Geometry: see drawing. Coordinates: mm, zero at the bounding-box minimum. A direction names the side the tool comes from. Give positions to 0.01 mm unless a question says otherwise; leave off trailing zeros. Order: outer loops, then holes, each group sorted by start corner. A loop starts at its lowest first (then second) coordinate and runs counter-clockwise, first axis right, second up. Notation, with made-up numbers: M 50.5,29 L 94.5,29 A8 cw 94.5,39 Z; hole C 63.5,-29 d4. An arc over 180 degrees is marked long. Return JSON: item names as keys, results as strings.
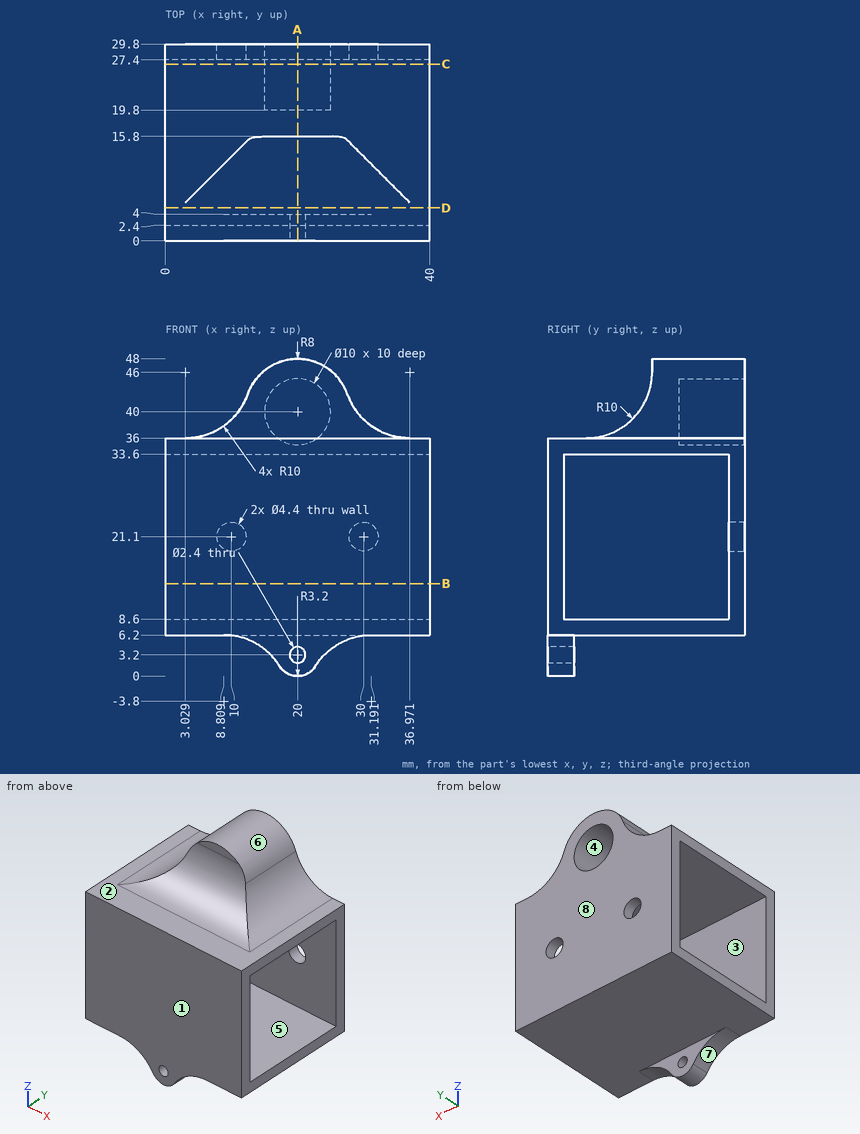
1. Section query A-A (x = 20). Return loops of the section in (y, z).
Evaluation:
{"outline": "M 0,0 L 4,0 L 4,2 L 0,2 Z; M 0,4.4 L 4,4.4 L 4,6.2 L 29.8,6.2 L 29.8,35 L 19.8,35 L 19.8,45 L 29.8,45 L 29.8,48 L 15.8,48 L 15.8,46 A10 cw 5.8,36 L 0,36 Z; hole M 2.4,8.6 L 27.4,8.6 L 27.4,33.6 L 2.4,33.6 Z"}
2. First-contact query: pin 1 (2 mm diameter, centred on x = 10.5, z = 39, fed in from -Y); pin 2 (15 mm diameter, centred on x = 11.5, y = 19.5, fed in from +Z); pin 3 (6 mm diameter, centred on x = 32, y = 16, fed in from -Z); pin 4 (5 mm diameter, centred on x = 32, z = 9, fed in from -Y). Flat tips, straight axial feed; report the tip coordinate or a pass-through.
Evaluation:
{"pin 1": "stops at y = 11.8", "pin 2": "stops at z = 47.94", "pin 3": "stops at z = 6.2", "pin 4": "stops at y = 0"}
3. Section query B-B (z = 14). Return loops of the section in (x, y).
Evaluation:
{"outline": "M 0,0 L 40,0 L 40,2.4 L 0,2.4 Z; M 0,27.4 L 40,27.4 L 40,29.8 L 0,29.8 Z"}
4. Ray query, probe 1 along X at (y, z) = (29.25, 21.1); probe 2 along Z at (x, y) = (20, 24.75); probe 3 along Z at (x, y) = (36.5, 3.75). Return the intervals inside material, ascending.
Evaluation:
{"probe 1": "x = 0 to 7.8, 12.2 to 27.8, 32.2 to 40", "probe 2": "z = 6.2 to 8.6, 33.6 to 35, 45 to 48", "probe 3": "z = 6.2 to 8.6, 33.6 to 36"}
5. Section query C-C (y = 26.75). Return loops of the section in (x, z), then the cut area to 3 significant figures.
Evaluation:
{"outline": "M 0,6.2 L 40,6.2 L 40,8.6 L 0,8.6 Z; M 0,33.6 L 40,33.6 L 40,36 L 36.97,36 A10 cw 27.54,42.67 A8 ccw 12.46,42.67 A10 cw 3.03,36 L 0,36 Z; hole C 20,40 d10", "area": "307 mm^2"}
6. Section query D-D (y = 5). Return loops of the section in (x, z).
Evaluation:
{"outline": "M 0,6.2 L 40,6.2 L 40,8.6 L 0,8.6 Z; M 0,33.6 L 40,33.6 L 40,36 L 0,36 Z"}
7. Set-up query: the marked faces 1, 2, 3 and 4. Return all of +Z, -Z, +X, -X, +Y, -Y with unobstructed straight access to the full face (end or side cutting, diameter ignored); none if empty.
Evaluation:
{"face 1": "+Z, -Z, +X, -X, -Y", "face 2": "+Z, -Y", "face 3": "+X, -X", "face 4": "+Y"}
8. Draft query along Z for the marked faces 5, 6, 7 and 8. Return one class per face: pulls with the +Z half, pulls with the -Z half, needs draft (parallel to the pull), parting line crosses it, or undercut.
Evaluation:
{"face 5": "undercut", "face 6": "pulls with the +Z half", "face 7": "pulls with the -Z half", "face 8": "needs draft"}
